Here's the drawing with two shaded views (mm, measured from the low corner). I have some questions. Round coordinates to 2 decimals unless told otherwise and drop trailing zeros. Loops run counter-clockwise (first coordinate to the right, second up) from the corner with the lowest first, then second, coordinate; pieces in that order, holes last.
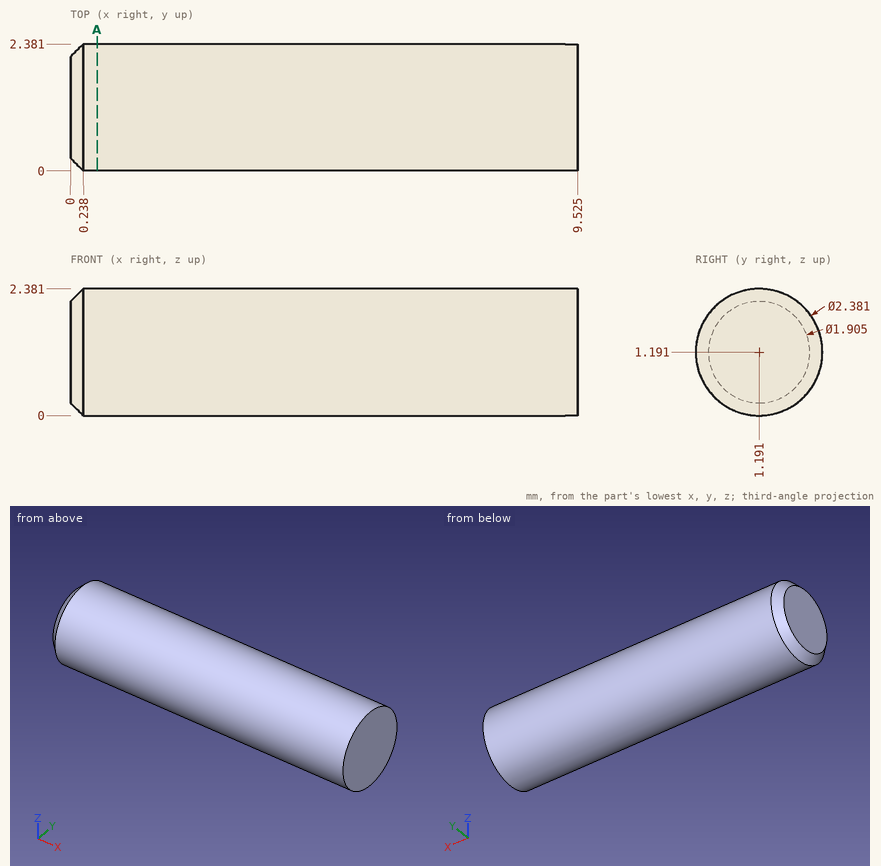
Item 1: Will this pin go through, and if not, where does the flat tip stop? pin 1 (1 mm diameter, centred on x = 1.5, y = 2, fed in from -Z).
Results list:
pin 1: stops at z = 0.04
Item 2: If I drill on line 1 along Z through (x, y) = (1, 1.25); line 2 along Y through (x, z) = (3.5, 0.25); line 3 along Z through (x, y) = (7.25, 1.95) (1 decimal), over which ranges is the centre line in solid material (lowest first)?
Results list:
line 1: z = 0 to 2.38
line 2: y = 0.46 to 1.92
line 3: z = 0.3 to 2.1
Item 3: If we section it at A-A, the plane x = 0.5: Please give me the cut outline in (y, z).
Results list:
outline: circle Ø2.38 at (1.19, 1.19)
